Verification items for the finished model (mm, model axes). Give positions to 0.01 mm unless a question says otherwise; leave off trailing zeros. Loops run counter-clockwise (first coordinate to the right, second up) from the corner with the lowest first, then second, coordinate; pieces in that order, holes last. Notation, with made-up numbers: (4, -2.75) - (10, -2.75) arc R24 cw to (10, 30.25) - close; hole circle Ø9 at (68, -35). An arc over 180 degrees is marked (long way). One line per question, with ' | ' between items. Start each with the question number.
1. Thickness scan on line 1 along X through (y, z) = (-1.3, 30); line 2 along X through (y, z) = (-1.7, 54); line 3 along Z through (x, y) = (-3, -1.2). Record the ranges inside material, lowest first. Write a range as from..to.
2. Section check A-A, the plane x = -27. State how many separate pieces and enclosed holes the cut face has, then the cut area to 3 significant figures.
3. Mould release check, pull along Z, two halves, no side actions. Record for faces 1 (the face through (7.833, -1.014, 39.027)), 2 (the face through (29, -1, 1)), 3 (the face through (-2.4, -1, 26.8)), 4 (the face through (-30, -1, 30)): +Z half, -Z half, draft (parallel to the pull), parting line (faces both ways), or undercut.
4. Section check C-C, the plane x = 0. Enter the section's corners in (y, z), then the cut area to 3 significant figures.
5. Section check D-D, the plane z = 30. Enter the section's corners in (x, y), then the cut area to 3 significant figures.
6. Section check B-B, the plane z = 56.5. Enter the section's corners in (x, y).
7. Depth check by flat-ended pin: pin 1 Ø13 at (x, z) = (0, 30) entering from +Y; pin 2 Ø4.5 at (x, z) = (27, 3.5) entering from -Y. Enter the tip coordinate at first touch or a pass-through.
from build123d import *

# Parameters (mm, degrees)
SKETCH1_W                                    = 60
SKETCH1_H                                    = 2
BASE_FLANGE1_DEPTH                           = 60
SKETCH2_R                                    = 1.25
CUT_EXTRUDE1_DEPTH                           = 10
CSK_FOR_M3_HEX_SOCKET_COUNTERSUNK_HE_2_COUNT = 2
CSK_FOR_M3_HEX_SOCKET_COUNTERSUNK_HE_2_PITCH = 54
CSK_FOR_M3_HEX_SOCKET_COUNTERSUNK_HE_3_COUNT = 2
CSK_FOR_M3_HEX_SOCKET_COUNTERSUNK_HE_3_PITCH = 53
CSK_FOR_M3_HEX_SOCKET_COUNTERSUNK_HE_4_COUNT = 2
CSK_FOR_M3_HEX_SOCKET_COUNTERSUNK_HE_4_PITCH = 75.663729752
CUT_EXTRUDE2_REACH                           = 69.112
SKETCH4_R                                    = 4
CHAMFER1_SIZE                                = 2
CUT_EXTRUDE3_REACH                           = 69.112
SKETCH5_R                                    = 1.25
SKETCH5_R_2                                  = 1


# Sheet-metal steps are written as plain solids
with BuildPart() as part:
    # Sketch1 → Base-Flange1 (new body)
    with BuildSketch(Plane.XY):
        with Locations((0, -1)):
            Rectangle(SKETCH1_W, SKETCH1_H)
    extrude(amount=BASE_FLANGE1_DEPTH)

    # Sketch2 → Cut-Extrude1 (cut)
    with BuildSketch(Plane(origin=(0, 0, 0), x_dir=(1, 0, 0), z_dir=(0, 1, 0))):
        with Locations(Location((-27, -3.5, 0), (0, 0, 270))):
            Circle(SKETCH2_R)
        with Locations(Location((-27, -56.5, 0), (0, 0, 270))):
            Circle(SKETCH2_R)
        with Locations(Location((27, -56.5, 0), (0, 0, 270))):
            Circle(SKETCH2_R)
        with Locations(Location((27, -3.5, 0), (0, 0, 270))):
            Circle(SKETCH2_R)
    extrude(amount=-CUT_EXTRUDE1_DEPTH, mode=Mode.SUBTRACT)

    # Sketch3 → CSK for M3 Hex Socket Countersunk Head Screw1 (revolve, cut)
    with BuildSketch(Plane(origin=(27, -2, 3.5), x_dir=(0, 0, -1), z_dir=(1, 0, 0))):
        Polygon((0, 0), (0, 2), (1.7, 2), (1.7, 1.77), (3.47, 0), align=None)
    csk_for_m3_hex_socket_countersunk_head_s = revolve(axis=Axis((27, -8.35, 3.5), (0, 1, 0)), mode=Mode.SUBTRACT)

    # CSK for M3 Hex Socket Countersunk He 2: CSK for M3 Hex Socket Countersunk Head Screw1 ×2
    with Locations(*[(-i * CSK_FOR_M3_HEX_SOCKET_COUNTERSUNK_HE_2_PITCH, 0, 0) for i in range(1, CSK_FOR_M3_HEX_SOCKET_COUNTERSUNK_HE_2_COUNT)]):
        add(csk_for_m3_hex_socket_countersunk_head_s, mode=Mode.SUBTRACT)

    # CSK for M3 Hex Socket Countersunk He 3: CSK for M3 Hex Socket Countersunk Head Screw1 ×2
    with Locations(*[(0, 0, i * CSK_FOR_M3_HEX_SOCKET_COUNTERSUNK_HE_3_PITCH) for i in range(1, CSK_FOR_M3_HEX_SOCKET_COUNTERSUNK_HE_3_COUNT)]):
        add(csk_for_m3_hex_socket_countersunk_head_s, mode=Mode.SUBTRACT)

    # CSK for M3 Hex Socket Countersunk He 4: CSK for M3 Hex Socket Countersunk Head Screw1 ×2
    with Locations(*[Vector(-0.7136840884914971, 0, 0.7004677164823951) * (i * CSK_FOR_M3_HEX_SOCKET_COUNTERSUNK_HE_4_PITCH) for i in range(1, CSK_FOR_M3_HEX_SOCKET_COUNTERSUNK_HE_4_COUNT)]):
        add(csk_for_m3_hex_socket_countersunk_head_s, mode=Mode.SUBTRACT)

    # Sketch4 → Cut-Extrude2 (cut, up to next)
    with BuildSketch(Plane(origin=(0, 0, 0), x_dir=(1, 0, 0), z_dir=(0, 1, 0)), mode=Mode.PRIVATE) as cut_extrude2_sk1:
        with Locations(Location((0, -30, 0), (0, 0, 270))):
            Circle(SKETCH4_R)
    cut_extrude2_tool1 = extrude(cut_extrude2_sk1.sketch, amount=-CUT_EXTRUDE2_REACH, mode=Mode.PRIVATE) & part.part
    add(cut_extrude2_tool1.solids().sort_by_distance((0, 0, 30))[0], mode=Mode.SUBTRACT)

    # Chamfer1
    # the kernel refuses this chamfer: 2 mm, written as the material it takes off along each edge
    with BuildSketch(Plane(origin=(30, 5.143365976, 0), x_dir=(-0.9996219169112968, 0, -0.02749587661058639), z_dir=(0, -1, 0)), Plane(origin=(-30, -7.143365976, 60), x_dir=(-0.027495876610585647, 0, -0.9996219169112968), z_dir=(0, 1, 0))) as chamfer1_piece_1:
        Polygon((CHAMFER1_SIZE * 0.999621916911, -CHAMFER1_SIZE * 0.0274958766106), (-CHAMFER1_SIZE * 0.0274958766106, -CHAMFER1_SIZE * 0.999621916911), (0, 0), align=None)
    extrude(amount=12.286731952, mode=Mode.SUBTRACT)
    with BuildSketch(Plane(origin=(30, 5.143365976, 60), x_dir=(-0.9996219169112968, 0, 0.027495876610585647), z_dir=(0, -1, 0)), Plane(origin=(-30, -7.143365976, 0), x_dir=(-0.02749587661058563, 0, 0.9996219169112968), z_dir=(0, 1, 0))) as chamfer1_piece_2:
        Polygon((CHAMFER1_SIZE * 0.999621916911, CHAMFER1_SIZE * 0.0274958766106), (-CHAMFER1_SIZE * 0.0274958766106, CHAMFER1_SIZE * 0.999621916911), (0, 0), align=None)
    extrude(amount=12.286731952, mode=Mode.SUBTRACT)

    # Sketch5 → Cut-Extrude3 (cut, up to next)
    with BuildSketch(Plane.XZ.offset(2), mode=Mode.PRIVATE) as cut_extrude3_sk1:
        with Locations(Location((7.778174593, 37.778174593, 0), (0, 0, 270))):
            Circle(SKETCH5_R)
    cut_extrude3_tool1 = extrude(cut_extrude3_sk1.sketch, amount=-CUT_EXTRUDE3_REACH, mode=Mode.PRIVATE) & part.part
    # Sketch5 → Cut-Extrude3 (cut, up to next)
    with BuildSketch(Plane.XZ.offset(2), mode=Mode.PRIVATE) as cut_extrude3_sk2:
        with Locations(Location((-7.778174593, 37.778174593, 0), (0, 0, 270))):
            Circle(SKETCH5_R)
    cut_extrude3_tool2 = extrude(cut_extrude3_sk2.sketch, amount=-CUT_EXTRUDE3_REACH, mode=Mode.PRIVATE) & part.part
    # Sketch5 → Cut-Extrude3 (cut, up to next)
    with BuildSketch(Plane.XZ.offset(2), mode=Mode.PRIVATE) as cut_extrude3_sk3:
        with Locations(Location((-7.778174593, 22.221825407, 0), (0, 0, 270))):
            Circle(SKETCH5_R)
    cut_extrude3_tool3 = extrude(cut_extrude3_sk3.sketch, amount=-CUT_EXTRUDE3_REACH, mode=Mode.PRIVATE) & part.part
    # Sketch5 → Cut-Extrude3 (cut, up to next)
    with BuildSketch(Plane.XZ.offset(2), mode=Mode.PRIVATE) as cut_extrude3_sk4:
        with Locations(Location((7.778174593, 22.221825407, 0), (0, 0, 270))):
            Circle(SKETCH5_R)
    cut_extrude3_tool4 = extrude(cut_extrude3_sk4.sketch, amount=-CUT_EXTRUDE3_REACH, mode=Mode.PRIVATE) & part.part
    # Sketch5 → Cut-Extrude3 (cut, up to next)
    with BuildSketch(Plane.XZ.offset(2), mode=Mode.PRIVATE) as cut_extrude3_sk5:
        with Locations(Location((8, 30, 0), (0, 0, 270))):
            Circle(SKETCH5_R_2)
    cut_extrude3_tool5 = extrude(cut_extrude3_sk5.sketch, amount=-CUT_EXTRUDE3_REACH, mode=Mode.PRIVATE) & part.part
    # Sketch5 → Cut-Extrude3 (cut, up to next)
    with BuildSketch(Plane.XZ.offset(2), mode=Mode.PRIVATE) as cut_extrude3_sk6:
        with Locations(Location((0, 22, 0), (0, 0, 270))):
            Circle(SKETCH5_R_2)
    cut_extrude3_tool6 = extrude(cut_extrude3_sk6.sketch, amount=-CUT_EXTRUDE3_REACH, mode=Mode.PRIVATE) & part.part
    # Sketch5 → Cut-Extrude3 (cut, up to next)
    with BuildSketch(Plane.XZ.offset(2), mode=Mode.PRIVATE) as cut_extrude3_sk7:
        with Locations(Location((-8, 30, 0), (0, 0, 270))):
            Circle(SKETCH5_R_2)
    cut_extrude3_tool7 = extrude(cut_extrude3_sk7.sketch, amount=-CUT_EXTRUDE3_REACH, mode=Mode.PRIVATE) & part.part
    # Sketch5 → Cut-Extrude3 (cut, up to next)
    with BuildSketch(Plane.XZ.offset(2), mode=Mode.PRIVATE) as cut_extrude3_sk8:
        with Locations(Location((0, 38, 0), (0, 0, 270))):
            Circle(SKETCH5_R_2)
    cut_extrude3_tool8 = extrude(cut_extrude3_sk8.sketch, amount=-CUT_EXTRUDE3_REACH, mode=Mode.PRIVATE) & part.part
    add(cut_extrude3_tool1.solids().sort_by_distance((7.778175, -2, 37.778175))[0], mode=Mode.SUBTRACT)
    add(cut_extrude3_tool2.solids().sort_by_distance((-7.778175, -2, 37.778175))[0], mode=Mode.SUBTRACT)
    add(cut_extrude3_tool3.solids().sort_by_distance((-7.778175, -2, 22.221825))[0], mode=Mode.SUBTRACT)
    add(cut_extrude3_tool4.solids().sort_by_distance((7.778175, -2, 22.221825))[0], mode=Mode.SUBTRACT)
    add(cut_extrude3_tool5.solids().sort_by_distance((8, -2, 30))[0], mode=Mode.SUBTRACT)
    add(cut_extrude3_tool6.solids().sort_by_distance((0, -2, 22))[0], mode=Mode.SUBTRACT)
    add(cut_extrude3_tool7.solids().sort_by_distance((-8, -2, 30))[0], mode=Mode.SUBTRACT)
    add(cut_extrude3_tool8.solids().sort_by_distance((0, -2, 38))[0], mode=Mode.SUBTRACT)


solid = part.part
Results list:
1) line 1: -30..-9, -7..-4, 4..7, 9..30 | line 2: -30..-28.95, -25.05..25.05, 28.95..30 | line 3: 0..27.35, 32.65..60
2) separate pieces: 3 | enclosed holes: 0 | area: 100 mm²
3) face 1: undercut | face 2: -Z half | face 3: undercut | face 4: draft
4) outline: (-2, 0) - (0, 0) - (0, 21) - (-2, 21) - close; (-2, 23) - (0, 23) - (0, 26) - (-2, 26) - close; (-2, 34) - (0, 34) - (0, 37) - (-2, 37) - close; (-2, 39) - (0, 39) - (0, 60) - (-2, 60) - close | area: 96.0 mm²
5) outline: (-30, -2) - (-9, -2) - (-9, 0) - (-30, 0) - close; (-7, -2) - (-4, -2) - (-4, 0) - (-7, 0) - close; (4, -2) - (7, -2) - (7, 0) - (4, 0) - close; (9, -2) - (30, -2) - (30, 0) - (9, 0) - close | area: 96.0 mm²
6) outline: (-30, -1.53) - (-28.7, -0.23) - (-28.7, 0) - (-30, 0) - close; (-25.3, -0.23) - (-23.53, -2) - (23.53, -2) - (25.3, -0.23) - (25.3, 0) - (-25.3, 0) - close; (28.7, -0.23) - (30, -1.53) - (30, 0) - (28.7, 0) - close
7) pin 1: y = 0 | pin 2: y = -0.78
